Can you work these out from the model? Positions are in its coordinate system, mm. A direction names the side the tool comes from. Give positions to 0.01 mm unless a question says otherwise; leave off trailing zeros. Order: outer loops, then holes, each group sorted by start corner. A loop starts at its lowest first (then second) coordinate and runs counter-clockwise, first axis right, second up. Notation, with made-up numbers: (-1, -11.5) - (7, -11.5) arc R21 ccw to (7, -3.5) - close; hole circle Ø2 at (26, -14.75). An arc over 180 degrees is marked (long way). Answer as CSV lines item,"result".
```python
from build123d import *

# Parameters (mm, degrees)
EXTRUDE_1_DEPTH                            = 12
EXTRUDE_1_2_DEPTH                          = 36
EXTRUDE_2_DEPTH                            = 8
EXTRUDE_3_DEPTH                            = 36
EXTRUDE_START                              = 56
EXTRUDE_4_DEPTH                            = 10
SKETCH_6_R                                 = 17.5
EXTRUDE_5_DEPTH                            = 20
CUT_EXTRUDE_1_REACH                        = 157.448
SKETCH_7_R                                 = 10
CUT_EXTRUDE_2_REACH                        = 157.448
HOLE_WIZARD_M16_1_D                        = 14
CUT_EXTRUDE_START                          = 10
CUT_EXTRUDE_3_DEPTH                        = 111.498756211
SKETCH_20_R                                = 6
CUT_EXTRUDE_4_DEPTH                        = 128.82800945
MIRROR_4_AT_THE_SECOND_PLANE_COPY_1_SKET_R = 6
MIRROR_4_AT_THE_SECOND_PLANE_COPY_1_DEPTH  = 128.82800945
CUT_EXTRUDE_5_DEPTH                        = 4


# Read off the part's stored shape, not the designer's step: the hole wizard step
with BuildPart() as part:
    # Sketch 1 → Extrude 1 (new body)
    with BuildSketch(Plane(origin=(0, 0, 0), x_dir=(1, 0, 0), z_dir=(0, 1, 0))):
        with BuildLine():
            Line((-46, -36), (46, -36))
            ThreePointArc((46, -36), (55.899494937, -31.899494937), (60, -22))
            Line((60, -22), (60, 22))
            ThreePointArc((60, 22), (55.899494937, 31.899494937), (46, 36))
            Line((46, 36), (-46, 36))
            ThreePointArc((-46, 36), (-55.899494937, 31.899494937), (-60, 22))
            Line((-60, 22), (-60, -22))
            ThreePointArc((-60, -22), (-55.899494937, -31.899494937), (-46, -36))
        make_face()
    extrude(amount=EXTRUDE_1_DEPTH)



with BuildPart() as body_2:
    # Sketch 2 → Extrude 1 2 (new, symmetric)
    with BuildSketch(Plane.XY):
        with BuildLine():
            Line((-31, 102), (0, 102))
            ThreePointArc((0, 102), (22, 80), (0, 58))
            Line((0, 58), (-31, 58))
            Line((-31, 58), (-31, 50))
            Line((-31, 50), (0, 50))
            ThreePointArc((0, 50), (30, 80), (0, 110))
            Line((0, 110), (-31, 110))
            Line((-31, 110), (-31, 102))
        make_face()
    extrude(amount=EXTRUDE_1_2_DEPTH, both=True)

    # Sketch 3 → Extrude 2 (add)
    with BuildSketch(Plane.XY.offset(36)):
        with BuildLine():
            Line((-31, 110), (-31, 50))
            Line((-31, 50), (0, 50))
            ThreePointArc((0, 50), (30, 80), (0, 110))
            Line((0, 110), (-31, 110))
        make_face()
    extrude_2 = extrude(amount=-EXTRUDE_2_DEPTH)

    # Mirror 1: Extrude 2 across plane
    add(extrude_2.mirror(Plane.XY))


with BuildPart() as part_1:
    add(part.part)

    add(body_2.part)  # Extrude 3 merges body 2
    # Sketch 4 → Extrude 3 (add, symmetric)
    with BuildSketch(Plane.XY):
        with BuildLine():
            Line((-25, 12), (-25, 50))
            Line((-25, 50), (0, 50))
            ThreePointArc((0, 50), (14.186371655, 53.566179631), (25, 63.416876048))
            Line((25, 63.416876048), (25, 12))
            Line((25, 12), (-25, 12))
        make_face()
    extrude(amount=EXTRUDE_3_DEPTH, both=True)



with BuildPart() as body_2_2:
    # Sketch 5 → Extrude 4 (new body)
    with BuildSketch(Plane.XY.offset(EXTRUDE_START)):
        with BuildLine():
            Line((15.407407407, 100.943060831), (32.925925926, 88.055023397))
            ThreePointArc((32.925925926, 88.055023397), (37, 80), (32.925925926, 71.944976603))
            Line((32.925925926, 71.944976603), (15.407407407, 59.056939169))
            ThreePointArc((15.407407407, 59.056939169), (0, 54), (-15.407407407, 59.056939169))
            Line((-15.407407407, 59.056939169), (-32.925925926, 71.944976603))
            ThreePointArc((-32.925925926, 71.944976603), (-37, 80), (-32.925925926, 88.055023397))
            Line((-32.925925926, 88.055023397), (-15.407407407, 100.943060831))
            ThreePointArc((-15.407407407, 100.943060831), (0, 106), (15.407407407, 100.943060831))
        make_face()
    extrude(amount=-EXTRUDE_4_DEPTH)


with BuildPart() as part_2:
    add(part_1.part)

    add(body_2_2.part)  # Extrude 5 merges body 2 2
    # Sketch 6 → Extrude 5 (add)
    with BuildSketch(Plane.XY.offset(56)):
        with Locations(Location((0, 80, 0), (0, 0, 180))):
            Circle(SKETCH_6_R)
    extrude(amount=-EXTRUDE_5_DEPTH)

    # Sketch 7 → Cut-Extrude 1 (cut, up to next)
    with BuildSketch(Plane.XY.offset(56), mode=Mode.PRIVATE) as cut_extrude_1_sk1:
        with Locations((0, 80)):
            Circle(SKETCH_7_R)
    cut_extrude_1_tool1 = extrude(cut_extrude_1_sk1.sketch, amount=-CUT_EXTRUDE_1_REACH, mode=Mode.PRIVATE) & part_2.part
    add(cut_extrude_1_tool1.solids().sort_by_distance((0, 80, 56))[0], mode=Mode.SUBTRACT)

    # Sketch 8 → Cut-Extrude 2 (cut, up to next)
    with BuildSketch(Plane.XY.offset(56), mode=Mode.PRIVATE) as cut_extrude_2_sk1:
        with BuildLine():
            Line((27, 84), (48.849510695, 84))
            ThreePointArc((48.849510695, 84), (52.849510695, 80), (48.849510695, 76))
            Line((48.849510695, 76), (27, 76))
            ThreePointArc((27, 76), (23, 80), (27, 84))
        make_face()
    cut_extrude_2_tool1 = extrude(cut_extrude_2_sk1.sketch, amount=-CUT_EXTRUDE_2_REACH, mode=Mode.PRIVATE) & part_2.part
    cut_extrude_2 = cut_extrude_2_tool1.solids().sort_by_distance((37.924755, 80, 56))[0]
    add(cut_extrude_2, mode=Mode.SUBTRACT)

    # Mirror 2: Cut-Extrude 2 across plane
    add(cut_extrude_2.mirror(Plane(origin=(0, 0, 0), x_dir=(0, 0, 1), z_dir=(1, 0, 0))), mode=Mode.SUBTRACT)

    # Hole Wizard M16 _1 (through all)
    with Locations(Plane.XY.offset(56)):
        with Locations((0, 80)):
            Hole(HOLE_WIZARD_M16_1_D / 2)

    # Hole Wizard M5 _1 outline → Hole Wizard M5 _1 (revolve, cut)
    with BuildSketch(Plane(origin=(0, 56, 30), x_dir=(0, 1, 0), z_dir=(0, 0, -1))):
        Polygon((2.1, -18.2618073), (0, -17), (0, -31), (2.1, -31), align=None)
    revolve(axis=Axis((0, 56, 30), (1, 0, 0)), mode=Mode.SUBTRACT)

    # Hole Wizard M5 _1 2 outline → Hole Wizard M5 _1 2 (revolve, cut)
    with BuildSketch(Plane(origin=(0, 104, -30), x_dir=(0, 1, 0), z_dir=(0, 0, -1))):
        Polygon((2.1, -18.2618073), (0, -17), (0, -31), (2.1, -31), align=None)
    revolve(axis=Axis((0, 104, -30), (1, 0, 0)), mode=Mode.SUBTRACT)

    # Hole Wizard M5 _1 3 outline → Hole Wizard M5 _1 3 (revolve, cut)
    with BuildSketch(Plane(origin=(0, 56, -30), x_dir=(0, 1, 0), z_dir=(0, 0, -1))):
        Polygon((2.1, -18.2618073), (0, -17), (0, -31), (2.1, -31), align=None)
    revolve(axis=Axis((0, 56, -30), (1, 0, 0)), mode=Mode.SUBTRACT)

    # Hole Wizard M5 _1 4 outline → Hole Wizard M5 _1 4 (revolve, cut)
    with BuildSketch(Plane(origin=(0, 104, 30), x_dir=(0, 1, 0), z_dir=(0, 0, -1))):
        Polygon((2.1, -18.2618073), (0, -17), (0, -31), (2.1, -31), align=None)
    revolve(axis=Axis((0, 104, 30), (1, 0, 0)), mode=Mode.SUBTRACT)

    # Sketch 15 → Cut-Extrude 3 (cut, through all)
    with BuildSketch(Plane(origin=(0, 58, 0), x_dir=(1, 0, 0), z_dir=(0, 1, 0)).offset(CUT_EXTRUDE_START)):
        with BuildLine():
            Line((-6, -6), (-6, 6))
            ThreePointArc((-6, 6), (0, 12), (6, 6))
            Line((6, 6), (6, -6))
            ThreePointArc((6, -6), (0, -12), (-6, -6))
        make_face()
    extrude(amount=-CUT_EXTRUDE_3_DEPTH, mode=Mode.SUBTRACT)

    # Sketch 17 → Hole Wizard 1 (revolve, cut)
    with BuildSketch(Plane(origin=(0, 30, 36), x_dir=(0, -1, 0), z_dir=(1, 0, 0))):
        Polygon((0, 0), (0, 60.407745571), (9, 55), (9, 18.403442476), (13, 16), (13, 0), align=None)
    revolve(axis=Axis((0, 30, 42.130023899), (0, 0, -1)), mode=Mode.SUBTRACT)

    # Sketch 19 → Hole Wizard M6 _1 (revolve, cut)
    with BuildSketch(Plane(origin=(-19, 30, 36), x_dir=(0, -1, 0), z_dir=(1, 0, 0))):
        Polygon((0, 0), (0, 17.502151548), (2.5, 16), (2.5, 0.525), (3.025, 0), align=None)
    hole_wizard_m6_1 = revolve(axis=Axis((-19, 30, 42.35), (0, 0, -1)), mode=Mode.SUBTRACT)

    # Mirror 3: Hole Wizard M6 _1 across plane
    add(hole_wizard_m6_1.mirror(Plane(origin=(0, 0, 0), x_dir=(0, 0, 1), z_dir=(1, 0, 0))), mode=Mode.SUBTRACT)

    # Sketch 20 → Cut-Extrude 4 (cut, through all)
    with BuildSketch(Plane(origin=(0, 12, 0), x_dir=(1, 0, 0), z_dir=(0, 1, 0))):
        with Locations(Location((-46, 22, 0), (0, 0, 270))):
            Circle(SKETCH_20_R)
    cut_extrude_4 = extrude(amount=-CUT_EXTRUDE_4_DEPTH, mode=Mode.SUBTRACT)

    # Mirror 4: Cut-Extrude 4 across plane
    add(cut_extrude_4.mirror(Plane(origin=(0, 0, 0), x_dir=(0, 0, 1), z_dir=(1, 0, 0))), mode=Mode.SUBTRACT)

    # Mirror 4 at the second plane: Cut-Extrude 4 across plane
    add(cut_extrude_4.mirror(Plane.XY), mode=Mode.SUBTRACT)

    # Mirror 4 at the second plane copy 1 sket → Mirror 4 at the second plane copy 1 (cut, through all)
    with BuildSketch(Plane(origin=(0, 12, 0), x_dir=(-1, 0, 0), z_dir=(0, 1, 0))):
        with Locations(Location((-46, 22, 0), (0, 0, 270))):
            Circle(MIRROR_4_AT_THE_SECOND_PLANE_COPY_1_SKET_R)
    extrude(amount=-MIRROR_4_AT_THE_SECOND_PLANE_COPY_1_DEPTH, mode=Mode.SUBTRACT)

    # Sketch 21 → Cut-Extrude 5 (cut)
    with BuildSketch(Plane.XZ):
        with BuildLine():
            Line((-32.143593539, -24), (32.143593539, -24))
            ThreePointArc((32.143593539, -24), (36.100505063, -12.100505063), (48, -8.143593539))
            Line((48, -8.143593539), (48, 8.143593539))
            ThreePointArc((48, 8.143593539), (36.100505063, 12.100505063), (32.143593539, 24))
            Line((32.143593539, 24), (-32.143593539, 24))
            ThreePointArc((-32.143593539, 24), (-36.100505063, 12.100505063), (-48, 8.143593539))
            Line((-48, 8.143593539), (-48, -8.143593539))
            ThreePointArc((-48, -8.143593539), (-36.100505063, -12.100505063), (-32.143593539, -24))
        make_face()
    extrude(amount=-CUT_EXTRUDE_5_DEPTH, mode=Mode.SUBTRACT)


solid = part_2.part
```
1) I need wall thicknesses on line 1 along Z through (x, y) = (19.5, 81); line 2 along X through (y, z) = (30, 32); line 3 along X through (y, z) = (8, 22). Which ranges of each line are inside material? Lowest first, please. Write a range as [from, to].
Answer block:
line 1,"[-36, -28], [28, 36], [46, 56]"
line 2,"[-25, -21.5], [-16.5, -13], [13, 16.5], [21.5, 25]"
line 3,"[-60, -52], [-40, 40], [52, 60]"
2) I'm going to push flat-ended pins straight in: P1, Ø13, axis at y = 52, z = 1, coming from the -X side; P2, Ø1.5, axis at y = 50.5, z = 13.5, coming from the +X side; P3, Ø8.5, axis at x = 0, y = 80, coming from the +Z side; P4, Ø4.5, axis at x = -19, y = 30, coming from the +Z side. Where does each tip first touch, or does it pass through?
Answer block:
P1,"x = -31"
P2,"x = 25"
P3,"through"
P4,"z = 19.85"
3) I want a section at C-C on y = 45.5. Write out the boundary of the cut face in (x, z), plus the area to 3 significant figures.
Answer block:
outline,"(-25, -36) - (25, -36) - (25, 36) - (-25, 36) - close; hole (-6, -6) arc R6 ccw to (6, -6) - (6, 6) arc R6 ccw to (-6, 6) - close"
area,"3,340 mm2"
4) Which directions (+Z, -Z, +X, -X, +Y, -Y) give clear straight access to the entire face, cutting with the end or side of a thin tool? Please do faces 1 (the flat face through (17, 86, 46)), 2 (the cylindrical face through (-8.923, 31.172, -0.446)), 3 (the flat face through (-11, 80, -28)), 4 (the flat face through (0, 2, 24)).
Answer block:
face 1,"none"
face 2,"+Z"
face 3,"-X"
face 4,"-Y"
5) I want a section at B-B on z = -10.5. Write out the boundary of the cut face in (x, y).
Answer block:
outline,"(-60, 0) - (-38.02, 0) - (-38.02, 4) - (-3.97, 4) - (-3.97, 21.92) arc R9 cw to (-3.97, 38.08) - (-3.97, 58) - (-31, 58) - (-31, 50) - (-25, 50) - (-25, 12) - (-60, 12) - close; (-31, 102) - (0, 102) arc R22 cw to (3.97, 58.36) - (3.97, 38.08) arc R9 cw to (3.97, 21.92) - (3.97, 4) - (38.02, 4) - (38.02, 0) - (60, 0) - (60, 12) - (25, 12) - (25, 63.42) arc R30 ccw to (0, 110) - (-31, 110) - close"
6) If we mould it in two halves opening along Y, with no side actions, what happens to faces 5 (the flat face through (-6, 48, 0)), 6 (the cylindrical face through (35, 86, 51)), 7 (the flat face through (-16, 102, 0))? For each: +Y half, -Y half, draft (parallel to the pull), parting line (faces both ways), or undercut.
Answer block:
face 5,"draft"
face 6,"+Y half"
face 7,"undercut"
7) I want a section at A-A on y = 80. Write out the boundary of the cut face in (x, z), plus the area to 3 significant figures.
Answer block:
outline,"(-31, -36) - (-7, -36) - (-7, -28) - (-31, -28) - close; (-31, 28) - (-10, 28) - (-10, 56) - (-23, 56) - (-23, 46) - (-17.5, 46) - (-17.5, 36) - (-31, 36) - close; (7, -36) - (30, -36) - (30, 36) - (17.5, 36) - (17.5, 46) - (23, 46) - (23, 56) - (10, 56) - (10, 28) - (22, 28) - (22, -28) - (7, -28) - close"
area,"1,560 mm2"
